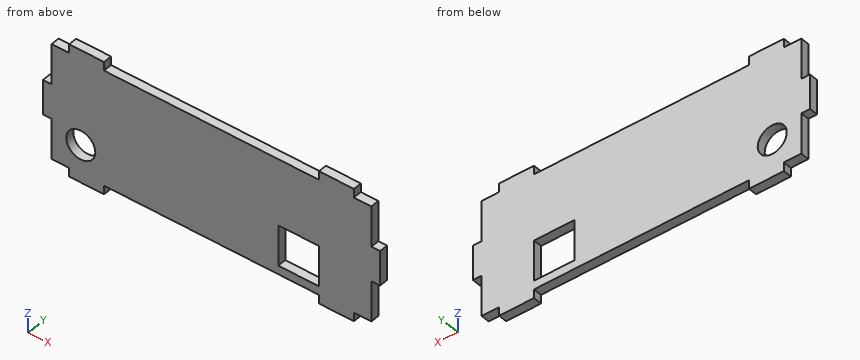
from build123d import *

# Parameters (mm, degrees)
F0_R     = 5
F0_W     = 14
F0_H     = 14
F1_DEPTH = 3


with BuildPart() as f1:
    # F0 (on Front) → F1 (new body)
    with BuildSketch(Plane.XZ):
        Polygon((55, 6), (55, 20), (49, 20), (49, 23), (37, 23), (37, 20), (-37, 20), (-37, 23), (-49, 23), (-49, 20), (-55, 20), (-55, 6), (-58, 6), (-58, -6), (-55, -6), (-55, -20), (-49, -20), (-49, -23), (-37, -23), (-37, -20), (37, -20), (37, -23), (49, -23), (49, -20), (55, -20), (55, -6), (58, -6), (58, 6), align=None)
        with Locations((-45, -10)):
            Circle(F0_R, mode=Mode.SUBTRACT)
        with Locations((30, -10)):
            Rectangle(F0_W, F0_H, mode=Mode.SUBTRACT)
    extrude(amount=F1_DEPTH)


solid = f1.part
CAD build for the part. Positions are in the model's coordinates, mm. Round coordinates to 2 decimals unless told otherwise and drop trailing zeros. Loops run counter-clockwise (first coordinate to the right, second up) from the corner with the lowest first, then second, coordinate; pieces in that order, holes last. Notation, with made-up numbers: M 28.25,-11 L 77.25,-11 A34 cw 77.25,21 Z; hole C -5,-21 d11. An arc over 180 degrees is marked long. One line per question, with ' | ' between items. Start each with the question number.
Item 1: Pin check, flat tips, straight feed: pin 1 Ø0.9 at (x, y) = (-52.5, -2) entering from +Z; pin 2 Ø1.5 at (y, z) = (-2, -6.5) entering from +X; pin 3 Ø0.9 at (y, z) = (-1, 22) entering from +X; pin 4 Ø0.9 at (x, y) = (57, -2) entering from +Z. Stop position of each tip, or through.
Item 2: Cut at B-B, the plane x = 27. Write the cut outline in (y, z), plus the area to 3 significant figures.
Item 3: Cut at D-D, the plane x = -45. Write the cut outline in (y, z).
Item 4: Wall check: line 1 (Z direction, x = -45, y = -1.45); line 2 (X direction, y = -2, z = -7); line 3 (Z direction, x = -52, y = -2.65). Give the ranges that are in metal, low to high.
Item 5: Cut at C-C, the plane y = -1.05. State how many separate pieces and enclosed holes the cut face has, plus the area to 3 significant figures.
Item 6: Cut at A-A, the plane z = -10. Write the cut outline in (x, y), plus the area to 3 significant figures.
Responses:
1) pin 1: stops at z = 20 | pin 2: stops at x = 58 | pin 3: stops at x = 49 | pin 4: stops at z = 6
2) outline: M -3,-20 L 0,-20 L 0,-17 L -3,-17 Z; M -3,-3 L 0,-3 L 0,20 L -3,20 Z | area: 78.0 mm²
3) outline: M -3,-23 L 0,-23 L 0,-15 L -3,-15 Z; M -3,-5 L 0,-5 L 0,23 L -3,23 Z
4) line 1: z = -23 to -15, -5 to 23 | line 2: x = -55 to -49, -41 to 23, 37 to 55 | line 3: z = -20 to 20
5) separate pieces: 1 | enclosed holes: 2 | area: 4,340 mm²
6) outline: M -55,-3 L -50,-3 L -50,0 L -55,0 Z; M -40,-3 L 23,-3 L 23,0 L -40,0 Z; M 37,-3 L 55,-3 L 55,0 L 37,0 Z | area: 258 mm²
